Part print with two shaded views. Sizes in mm from the minimum x, y, z corner. Round coordinates to 2 decimals unless told otherwise and drop trailing zeros. Loops run counter-clockwise (first coordinate to the right, second up) from the corner with the lowest first, then second, coordinate; pieces in that order, holes last. Notation, with made-up numbers: M 0.5,-21 L 57.5,-21 A21 cw 57.5,7 Z; hole C 80.5,36 d9. An arc over 180 degrees is marked long. Use a Markdown table: item, result. Add a question column.
Item 1: Saw through at B-B on z = 47.5. Write the cut outline in (x, y), then the cut area to 3 significant figures.
Item 2: Wall check: L1, parallel to Y at x = 11, z = 46 (1 decimal); L2, parallel to Y at x = 18.5, z = 36.5; L3, parallel to Z at x = 1, y = 76.5. Give the ranges that are in metal, low to high. Write a range as from..to.
Item 3: Pin check, flat tips, straight feed: P1, Ø3, axis at x = 9, y = 68.5, coming from the -Z side; P2, Ø8, axis at x = 7.5, z = 8.5, coming from the -Y side; P3, Ø3, axis at x = 22.5, y = 93.5, coming from the -Z side. Stop position of each tip, or through.
Item 4: Saw through at C-C on y = 116. Write the cut outline in (x, z).
Item 5: Saw through at A-A on x = 6.5. Write the cut outline in (y, z) (1 decimal).
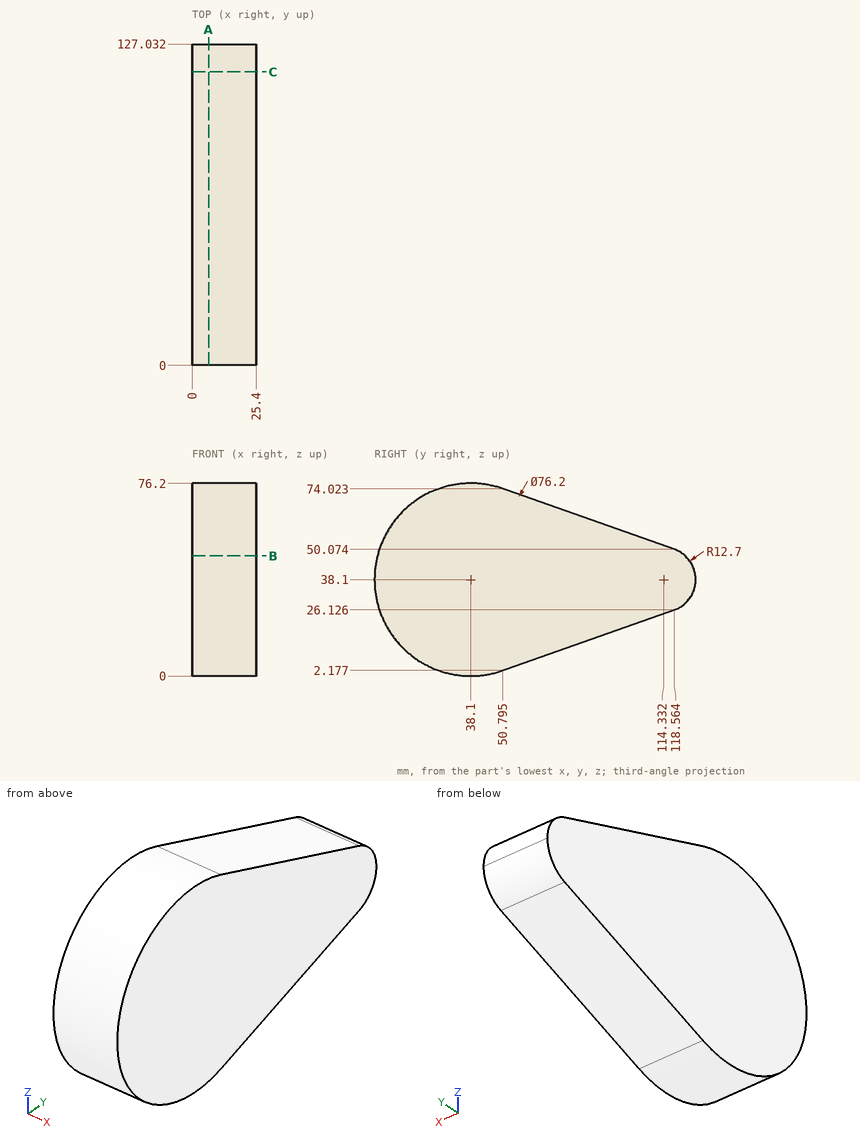
Entries:
| question | item | result |
|---|---|---|
| 1 | outline | M 0,1.18 L 25.4,1.18 L 25.4,122.87 L 0,122.87 Z |
| 1 | area | 3,090 mm2 |
| 2 | L1 | 0.8..124.3 |
| 2 | L2 | 0.03..126.93 |
| 2 | L3 | 11.26..64.94 |
| 3 | P1 | z = 7.9 |
| 3 | P2 | y = 9.88 |
| 3 | P3 | z = 16.74 |
| 4 | outline | M 0,25.22 L 25.4,25.22 L 25.4,50.98 L 0,50.98 Z |
| 5 | outline | M 50.8,2.2 L 118.6,26.1 A12.7 ccw 118.6,50.1 L 50.8,74 A38.1 ccw long Z |
